```python
from build123d import *

# Parameters (mm, degrees)
SKETCH1_W                                        = 300
SKETCH1_H                                        = 185
BOSS_EXTRUDE1_DEPTH                              = 38
CUT_EXTRUDE1_REACH                               = 243.183
SKETCH2_R                                        = 31.5
SKETCH3_R                                        = 55
CUT_EXTRUDE2_DEPTH                               = 22
CUT_EXTRUDE3_DEPTH                               = 10.8
CBORE_FOR_M10_SOCKET_HEAD_CAP_SCREW1_D           = 12
CBORE_FOR_M10_SOCKET_HEAD_CAP_SCREW1_CBORE_D     = 17.5
CBORE_FOR_M10_SOCKET_HEAD_CAP_SCREW1_CBORE_DEPTH = 10.8
LPATTERN1_COUNT                                  = 3
LPATTERN1_PITCH                                  = 45
M10X1_5_TAPPED_HOLE1_D                           = 8.5
M10X1_5_TAPPED_HOLE1_DEPTH                       = 24.5
M10X1_5_TAPPED_HOLE1_TIP                         = 2.553657631
M10X1_5_TAPPED_HOLE2_D                           = 8.5
M10X1_5_TAPPED_HOLE2_DEPTH                       = 24.5
M10X1_5_TAPPED_HOLE2_TIP                         = 2.553657631
M8X1_25_TAPPED_HOLE1_D                           = 6.8
M6X1_0_TAPPED_HOLE1_D                            = 5
M6X1_0_TAPPED_HOLE1_DEPTH                        = 15
M6X1_0_TAPPED_HOLE1_TIP                          = 1.502151548
M6X1_0_TAPPED_HOLE2_AT_2_COUNT                   = 2
M6X1_0_TAPPED_HOLE2_AT_2_PITCH                   = 26
M6X1_0_TAPPED_HOLE2_AT_3_COUNT                   = 2
M6X1_0_TAPPED_HOLE2_AT_3_PITCH                   = 93.680307429
M6X1_0_TAPPED_HOLE2_AT_4_COUNT                   = 2
M6X1_0_TAPPED_HOLE2_AT_4_PITCH                   = 90
M6X1_0_TAPPED_HOLE3_AT_2_COUNT                   = 2
M6X1_0_TAPPED_HOLE3_AT_2_PITCH                   = 125
M6X1_0_TAPPED_HOLE3_AT_3_COUNT                   = 2
M6X1_0_TAPPED_HOLE3_AT_3_PITCH                   = 250
LPATTERN3_COUNT                                  = 2
LPATTERN3_PITCH                                  = 26
CHAMFER1_SIZE                                    = 5
CHAMFER2_SIZE                                    = 1


with BuildPart() as part:
    # Sketch1 → Boss-Extrude1 (new body)
    with BuildSketch(Plane(origin=(0, 0, 0), x_dir=(1, 0, 0), z_dir=(0, 1, 0))):
        with Locations((0, -92.5)):
            Rectangle(SKETCH1_W, SKETCH1_H)
    extrude(amount=BOSS_EXTRUDE1_DEPTH)

    # Sketch2 → Cut-Extrude1 (cut, up to next)
    with BuildSketch(Plane(origin=(0, 38, 0), x_dir=(1, 0, 0), z_dir=(0, 1, 0)), mode=Mode.PRIVATE) as cut_extrude1_sk1:
        with Locations(Location((0, -85, 0), (0, 0, 270))):
            Circle(SKETCH2_R)
    cut_extrude1_tool1 = extrude(cut_extrude1_sk1.sketch, amount=-CUT_EXTRUDE1_REACH, mode=Mode.PRIVATE) & part.part
    add(cut_extrude1_tool1.solids().sort_by_distance((0, 38, 85))[0], mode=Mode.SUBTRACT)

    # Sketch3 → Cut-Extrude2 (cut)
    with BuildSketch(Plane(origin=(0, 38, 0), x_dir=(1, 0, 0), z_dir=(0, 1, 0))):
        with Locations(Location((0, -85, 0), (0, 0, 270))):
            Circle(SKETCH3_R)
    extrude(amount=-CUT_EXTRUDE2_DEPTH, mode=Mode.SUBTRACT)

    # Sketch6 → Cut-Extrude3 (cut)
    with BuildSketch(Plane(origin=(0, 38, 0), x_dir=(1, 0, 0), z_dir=(0, 1, 0))):
        with BuildLine():
            Line((-113.75, -8), (-113.75, 0))
            Line((-113.75, 0), (-96.25, 0))
            Line((-96.25, 0), (-96.25, -8))
            ThreePointArc((-96.25, -8), (-105, -16.75), (-113.75, -8))
        make_face()
        with BuildLine():
            Line((96.25, -8), (96.25, 0))
            Line((96.25, 0), (113.75, 0))
            Line((113.75, 0), (113.75, -8))
            ThreePointArc((113.75, -8), (105, -16.75), (96.25, -8))
        make_face()
    extrude(amount=-CUT_EXTRUDE3_DEPTH, mode=Mode.SUBTRACT)

    # CBORE for M10 Socket Head Cap Screw1 (through all)
    with Locations(Plane(origin=(0, 38, 0), x_dir=(-1, 0, 0), z_dir=(0, 1, 0))):
        with Locations((105, 8), (-105, 8)):
            cbore_for_m10_socket_head_cap_screw1 = CounterBoreHole(CBORE_FOR_M10_SOCKET_HEAD_CAP_SCREW1_D / 2, CBORE_FOR_M10_SOCKET_HEAD_CAP_SCREW1_CBORE_D / 2, CBORE_FOR_M10_SOCKET_HEAD_CAP_SCREW1_CBORE_DEPTH)

    # LPattern1: CBORE for M10 Socket Head Cap Screw1 ×3
    with Locations(*[(0, 0, i * LPATTERN1_PITCH) for i in range(1, LPATTERN1_COUNT)]):
        add(cbore_for_m10_socket_head_cap_screw1, mode=Mode.SUBTRACT)

    # M10x1.5 Tapped Hole1
    with Locations(Plane(origin=(0, 38, 0), x_dir=(-1, 0, 0), z_dir=(0, 1, 0))):
        with Locations((88, 8), (-88, 8), (-88, 117), (88, 117)):
            Hole(M10X1_5_TAPPED_HOLE1_D / 2, depth=M10X1_5_TAPPED_HOLE1_DEPTH)
            with Locations((0, 0, -(M10X1_5_TAPPED_HOLE1_DEPTH + M10X1_5_TAPPED_HOLE1_TIP / 2))):  # 118° drill point
                Cone(0, M10X1_5_TAPPED_HOLE1_D / 2, M10X1_5_TAPPED_HOLE1_TIP, mode=Mode.SUBTRACT)

    # M10x1.5 Tapped Hole2
    with Locations(Plane.XZ):
        with Locations((25, 174), (-25, 174)):
            Hole(M10X1_5_TAPPED_HOLE2_D / 2, depth=M10X1_5_TAPPED_HOLE2_DEPTH)
            with Locations((0, 0, -(M10X1_5_TAPPED_HOLE2_DEPTH + M10X1_5_TAPPED_HOLE2_TIP / 2))):  # 118° drill point
                Cone(0, M10X1_5_TAPPED_HOLE2_D / 2, M10X1_5_TAPPED_HOLE2_TIP, mode=Mode.SUBTRACT)

    # M8x1.25 Tapped Hole1 (through all)
    with Locations(Plane(origin=(0, 16, 0), x_dir=(-1, 0, 0), z_dir=(0, 1, 0))):
        with Locations((28.284271247, 113.284271247), (-28.284271247, 113.284271247), (-28.284271247, 56.715728753), (28.284271247, 56.715728753)):
            Hole(M8X1_25_TAPPED_HOLE1_D / 2)

    # M6x1.0 Tapped Hole1
    with Locations(Plane(origin=(0, 38, 0), x_dir=(-1, 0, 0), z_dir=(0, 1, 0))):
        with Locations((-71, 151), (71, 151), (-105, 151), (105, 151)):
            Hole(M6X1_0_TAPPED_HOLE1_D / 2, depth=M6X1_0_TAPPED_HOLE1_DEPTH)
            with Locations((0, 0, -(M6X1_0_TAPPED_HOLE1_DEPTH + M6X1_0_TAPPED_HOLE1_TIP / 2))):  # 118° drill point
                Cone(0, M6X1_0_TAPPED_HOLE1_D / 2, M6X1_0_TAPPED_HOLE1_TIP, mode=Mode.SUBTRACT)

    # Sketch15 → M6x1.0 Tapped Hole2 (revolve, cut)
    with BuildSketch(Plane(origin=(150, 6, 8), x_dir=(0, 0, -1), z_dir=(0, 1, 0))):
        Polygon((0, 0), (0, 16.502151548), (2.5, 15), (2.5, 0), align=None)
    m6x1_0_tapped_hole2 = revolve(axis=Axis((156.35, 6, 8), (-1, 0, 0)), mode=Mode.SUBTRACT)

    # M6x1.0 Tapped Hole2 at 2: M6x1.0 Tapped Hole2 ×2
    with Locations(*[(0, i * M6X1_0_TAPPED_HOLE2_AT_2_PITCH, 0) for i in range(1, M6X1_0_TAPPED_HOLE2_AT_2_COUNT)]):
        add(m6x1_0_tapped_hole2, mode=Mode.SUBTRACT)

    # M6x1.0 Tapped Hole2 at 3: M6x1.0 Tapped Hole2 ×2
    with Locations(*[Vector(0, 0.27753965282077453, 0.9607141828411425) * (i * M6X1_0_TAPPED_HOLE2_AT_3_PITCH) for i in range(1, M6X1_0_TAPPED_HOLE2_AT_3_COUNT)]):
        add(m6x1_0_tapped_hole2, mode=Mode.SUBTRACT)

    # M6x1.0 Tapped Hole2 at 4: M6x1.0 Tapped Hole2 ×2
    with Locations(*[(0, 0, i * M6X1_0_TAPPED_HOLE2_AT_4_PITCH) for i in range(1, M6X1_0_TAPPED_HOLE2_AT_4_COUNT)]):
        add(m6x1_0_tapped_hole2, mode=Mode.SUBTRACT)

    # Sketch17 → M6x1.0 Tapped Hole4 (revolve, cut)
    with BuildSketch(Plane(origin=(150, 32, 178), x_dir=(0, 0, -1), z_dir=(0, 1, 0))):
        Polygon((0, 0), (0, 16.502151548), (2.5, 15), (2.5, 0), align=None)
    m6x1_0_tapped_hole4 = revolve(axis=Axis((156.35, 32, 178), (-1, 0, 0)), mode=Mode.SUBTRACT)

    # Mirror1: M6x1.0 Tapped Hole2, M6x1.0 Tapped Hole4 across plane
    add(m6x1_0_tapped_hole2.mirror(Plane(origin=(0, 0, 0), x_dir=(0, 0, 1), z_dir=(1, 0, 0))), mode=Mode.SUBTRACT)
    add(m6x1_0_tapped_hole4.mirror(Plane(origin=(0, 0, 0), x_dir=(0, 0, 1), z_dir=(1, 0, 0))), mode=Mode.SUBTRACT)

    # Mirror1 copy 1 sketch → Mirror1 copy 1 (revolve, cut)
    with BuildSketch(Plane(origin=(-150, 32, 8), x_dir=(0, 0, -1), z_dir=(0, 1, 0))):
        Polygon((0, 0), (0, -16.502151548), (2.5, -15), (2.5, 0), align=None)
    revolve(axis=Axis((-156.35, 32, 8), (-1, 0, 0)), mode=Mode.SUBTRACT)

    # Mirror1 copy 2 sketch → Mirror1 copy 2 (revolve, cut)
    with BuildSketch(Plane(origin=(-150, 32, 98), x_dir=(0, 0, -1), z_dir=(0, 1, 0))):
        Polygon((0, 0), (0, -16.502151548), (2.5, -15), (2.5, 0), align=None)
    revolve(axis=Axis((-156.35, 32, 98), (-1, 0, 0)), mode=Mode.SUBTRACT)

    # Mirror1 copy 3 sketch → Mirror1 copy 3 (revolve, cut)
    with BuildSketch(Plane(origin=(-150, 6, 98), x_dir=(0, 0, -1), z_dir=(0, 1, 0))):
        Polygon((0, 0), (0, -16.502151548), (2.5, -15), (2.5, 0), align=None)
    revolve(axis=Axis((-156.35, 6, 98), (-1, 0, 0)), mode=Mode.SUBTRACT)

    # Sketch19 → M6x1.0 Tapped Hole3 (revolve, cut)
    with BuildSketch(Plane(origin=(125, 6, 185), x_dir=(0, -1, 0), z_dir=(1, 0, 0))):
        Polygon((0, 0), (0, 16.502151548), (2.5, 15), (2.5, 0), align=None)
    m6x1_0_tapped_hole3 = revolve(axis=Axis((125, 6, 191.35), (0, 0, -1)), mode=Mode.SUBTRACT)

    # M6x1.0 Tapped Hole3 at 2: M6x1.0 Tapped Hole3 ×2
    with Locations(*[(-i * M6X1_0_TAPPED_HOLE3_AT_2_PITCH, 0, 0) for i in range(1, M6X1_0_TAPPED_HOLE3_AT_2_COUNT)]):
        add(m6x1_0_tapped_hole3, mode=Mode.SUBTRACT)

    # M6x1.0 Tapped Hole3 at 3: M6x1.0 Tapped Hole3 ×2
    with Locations(*[(-i * M6X1_0_TAPPED_HOLE3_AT_3_PITCH, 0, 0) for i in range(1, M6X1_0_TAPPED_HOLE3_AT_3_COUNT)]):
        add(m6x1_0_tapped_hole3, mode=Mode.SUBTRACT)

    # LPattern3: M6x1.0 Tapped Hole3 ×2
    with Locations(*[(0, i * LPATTERN3_PITCH, 0) for i in range(1, LPATTERN3_COUNT)]):
        add(m6x1_0_tapped_hole3, mode=Mode.SUBTRACT)

    # LPattern3 copy 1 sketch → LPattern3 copy 1 (revolve, cut)
    with BuildSketch(Plane(origin=(0, 32, 185), x_dir=(0, -1, 0), z_dir=(1, 0, 0))):
        Polygon((0, 0), (0, 16.502151548), (2.5, 15), (2.5, 0), align=None)
    revolve(axis=Axis((0, 32, 191.35), (0, 0, -1)), mode=Mode.SUBTRACT)

    # LPattern3 copy 2 sketch → LPattern3 copy 2 (revolve, cut)
    with BuildSketch(Plane(origin=(-125, 32, 185), x_dir=(0, -1, 0), z_dir=(1, 0, 0))):
        Polygon((0, 0), (0, 16.502151548), (2.5, 15), (2.5, 0), align=None)
    revolve(axis=Axis((-125, 32, 191.35), (0, 0, -1)), mode=Mode.SUBTRACT)

    # Chamfer1
    # the kernel refuses this chamfer: 5 mm, written as the material it takes off along each edge
    with BuildSketch(Plane(origin=(150, -12.85841494, 185), x_dir=(0.027495876610587663, 0, -0.9996219169112968), z_dir=(0, 1, 0))) as chamfer1_piece_1:
        Polygon((CHAMFER1_SIZE * 0.999621916911, CHAMFER1_SIZE * 0.0274958766106), (-CHAMFER1_SIZE * 0.0274958766106, CHAMFER1_SIZE * 0.999621916911), (0, 0), align=None)
    extrude(amount=63.71682988, mode=Mode.SUBTRACT)
    with BuildSketch(Plane(origin=(-150, -12.85841494, 185), x_dir=(-0.027495876610587663, 0, -0.9996219169112968), z_dir=(0, 1, 0))) as chamfer1_piece_2:
        Polygon((CHAMFER1_SIZE * 0.999621916911, -CHAMFER1_SIZE * 0.0274958766106), (-CHAMFER1_SIZE * 0.0274958766106, -CHAMFER1_SIZE * 0.999621916911), (0, 0), align=None)
    extrude(amount=63.71682988, mode=Mode.SUBTRACT)

    # Chamfer2
    chamfer2_edges = [part.edges().sort_by_distance(p)[0] for p in [
        (0, 16, 53.5),
    ]]
    chamfer(chamfer2_edges, length=CHAMFER2_SIZE)


solid = part.part
```
Source: CAD feature listing. Evaluate the final solid. Frame: model axes, mm. A direction names the side the tool comes from. Give positions to 0.01 mm unless a question says otherwise; leave off trailing zeros. Loops run counter-clockwise (first coordinate to the right, second up) from the corner with the lowest first, then second, coordinate; pieces in that order, holes last. Notation, with made-up numbers: (69.25, -29) - (86.25, -29) arc R13 ccw to (86.25, -8) - close; hole circle Ø1 at (89, 1). An arc over 180 degrees is marked (long way). Use CSV: the item, a comma, the result in double quotes. Start each with the question number.
1. Pin query (flat end, axial travel): pin 1 (4.5 mm diameter, centred on y = 32, z = 8, fed in from -X); pin 2 (3 mm diameter, centred on y = 32, z = 98, fed in from +X); pin 3 (2 mm diameter, centred on x = 48.5, z = 61.5, fed in from +Y). Return the tip coordinate at first contact, or that it passes through.
2. Section A-A (z = 130.5). Output: boundary loops of the cut face in (x, y).
3. Draft query along Z for faces 1 (the flat face through (150, 19, 91)), 2 (the conical face through (-87.9, 11.39, 117.73)), 3 (the cylindrical face through (105.192, 32.676, 16.748)). Return one class per face: +Z half, -Z half, draft (parallel to the pull), parting line (faces both ways), or undercut.
4. Ray query, L1, parallel to Z at x = -105, y = 11; L2, parallel to Z at x = 88, y = 23; L3, parallel to Z at x = -142.25, y = 6. Return the intervals inside material, ascending.
5. Reachability of faces 4 (the flat face through (111, 27.2, 6)), 5 (the flat face through (-150, 19, 91)), 6 (the cylindrical face through (-96.26, 32.68, 53.38)), 7 (the cylindrical face through (25.553, 12.422, 178.214)), 8 (the cylindrical face through (27.547, 7.888, 109.965)) from +Z, -Z, +X, -X, +Y, -Y: full face, straight path, thin tool, end or side. Return the list, or none.
Response:
1,pin 1,"x = -134.85"
1,pin 2,"x = 134.4"
1,pin 3,"y = 16"
2,outline,"(-150, 0) - (150, 0) - (150, 38) - (30.9, 38) - (30.9, 16) - (-30.9, 16) - (-30.9, 38) - (-150, 38) - close"
3,face 1,"draft"
3,face 2,"undercut"
3,face 3,"-Z half"
4,L1,"0 to 2, 14 to 47, 59 to 92, 104 to 185"
4,L2,"0 to 3.75, 12.25 to 112.75, 121.25 to 185"
4,L3,"0 to 5.5, 10.5 to 95.5, 100.5 to 185"
5,face 4,"-Z, +Y"
5,face 5,"+Z, -Z, -X, +Y, -Y"
5,face 6,"+Y"
5,face 7,"-Y"
5,face 8,"+Y, -Y"
